Input: part model. Units: mm. Frame: model coordinates. A direction names the side the tool comes from. Round coordinates to 2 decimals unless told otherwise and drop trailing zeros. Loops run counter-clockwise (first coordinate to the right, second up) from the corner with the lowest first, then second, coordinate; pieces in that order, holes last. Notation, with made-up numbers: M -3.5,83.5 L 32.5,83.5 A31 ccw 32.5,119.5 Z; hole C 30,35 d10. An arc over 180 degrees is marked long. Put each result on its own line as item: value. Start each with the question number.
1) Pin query (flat end, axial travel): pin 1 (1.4 mm diameter, centred on x = -45.72, y = -33.02, fed in from +Z); pin 2 (3.5 mm diameter, centred on x = 45, y = 31.5, fed in from +Z); pin 3 (2.5 mm diameter, centred on x = -14.5, z = 28.5, fed in from -Y). Return the tip coordinate at first contact, or that it passes through.
2) Section C-C on z = 22.5. Output: boundary loops of the cut face in (x, y), plus the area to 3 significant figures.
3) Section B-B on z = 4. State how many separate pieces and enclosed holes the cut face has, plus the area to 3 significant figures.
4) Line query: probe 1 along Y at (x, z) = (-45.72, 3.2); probe 2 along Y at (x, z) = (4, 14.25); probe 3 along X at (y, z) = (-13.5, 11.5). Output: solid intervals per line, ascending.
5) Draft query along Z for faces 1 (the face through (-22.2, -41.23, 15.86)), 2 (the face through (52.5, 1, 9)), 3 (the face through (-1, 1, 0)), 4 (the face through (54, 0, 17)). Return one class per face: +Z half, -Z half, draft (parallel to the pull), parting line (faces both ways), or undercut.
6) Reachability of faces 5 (the face through (-1, 40, 14)), 6 (the face through (54, -12.7, 14)), 7 (the face through (-11, -41, 15)) from +Z, -Z, +X, -X, +Y, -Y: full face, straight path, thin tool, end or side. Return the list, or none.
7) Section D-D on x = -12.5. Output: boundary loops of the cut face in (y, z).
8) Section A-A on y = -7. Output: boundary loops of the cut face in (x, z), plus the area to 4 significant figures.
Autodesk Inventor part; units mm, degrees
ref_plane "YZ Plane" through (0, 0, 0) normal (1, 0, 0) x (0, 1, 0)
ref_plane "XZ Plane" through (0, 0, 0) normal (0, 1, 0) x (-1, 0, 0)
ref_plane "XY Plane" through (0, 0, 0) normal (0, 0, 1) x (1, 0, 0)
sketch "Esboço1" plane through (0, 0, 0) normal (0, 0, 1) x (1, 0, 0)
  line L0 (-55, -42.5) -> (55, -42.5)
  line L1 (55, -42.5) -> (55, 42.5)
  line L2 (55, 42.5) -> (-55, 42.5)
  line L3 (-55, 42.5) -> (-55, -42.5)
  line L4 (-55, -42.5) -> (55, 42.5) construction
  line L5 (55, -42.5) -> (-55, 42.5) construction
  point P0 (0, 0)
  dimension "d0" = 110
  dimension "d1" = 85
extrude "Extrusão1" add sketch "Esboço1" along normal blind 2
sketch "Esboço2" plane through (0, 0, 2) normal (0, 0, 1) x (1, 0, 0)
  line L0 (55, 42.5) -> (-55, 42.5)
  line L1 (55, -42.5) -> (-55, -42.5)
  line L2 (-55, -42.5) -> (-55, 42.5)
  line L3 (-55, 42.5) -> (55, 42.5)
  line L4 (55, 42.5) -> (55, -42.5)
  line L5 (55, -42.5) -> (-55, 42.5) construction
  line L6 (-55, -42.5) -> (55, 42.5) construction
  line L7 (52.5, -40) -> (-52.5, -40)
  line L8 (-52.5, -40) -> (-52.5, 40)
  line L9 (-52.5, 40) -> (52.5, 40)
  line L10 (52.5, 40) -> (52.5, -40)
  line L11 (52.5, -40) -> (-52.5, 40) construction
  line L12 (-52.5, -40) -> (52.5, 40) construction
  point P0 (0, 0)
  point P1 (55, 42.5)
  dimension "d4" = 105
  dimension "d5" = 80
extrude "Extrusão2" add sketch "Esboço2" along normal blind 25
sketch "Esboço3" plane through (0, 0, 2) normal (0, 0, 1) x (1, 0, 0)
  line L0 (-45.72, -33.02) -> (45.72, 33.02) construction
  line L1 (45.72, -33.02) -> (-45.72, 33.02) construction
  circle A0 centre (-45.72, 33.02) radius 3.5
  circle A1 centre (45.72, 33.02) radius 3.5
  circle A2 centre (-45.72, -33.02) radius 3.5
  circle A3 centre (45.72, -33.02) radius 3.5
  circle A4 centre (-45.72, 33.02) radius 0.75
  circle A5 centre (45.72, 33.02) radius 0.75
  circle A6 centre (-45.72, -33.02) radius 0.75
  circle A7 centre (45.72, -33.02) radius 0.75
  point P0 (0, 0)
  dimension "d10" = 7
  dimension "d11" = 7
  dimension "d12" = 7
  dimension "d13" = 7
  dimension "d20" = 1.5
  dimension "d21" = 1.5
  dimension "d22" = 1.5
  dimension "d23" = 1.5
extrude "Extrusão3" add sketch "Esboço3" along normal blind 5
sketch "Esboço4" plane through (0, 0, 27) normal (0, 0, 1) x (1, 0, 0)
  line L0 (55, -42.5) -> (-55, -42.5)
  line L1 (-55, -42.5) -> (-55, 42.5)
  line L2 (-55, 42.5) -> (55, 42.5)
  line L3 (55, 42.5) -> (55, -42.5)
  line L4 (55, -42.5) -> (-55, 42.5) construction
  line L5 (-55, -42.5) -> (55, 42.5) construction
  line L6 (54, -41.5) -> (-54, -41.5)
  line L7 (-54, -41.5) -> (-54, 41.5)
  line L8 (-54, 41.5) -> (54, 41.5)
  line L9 (54, 41.5) -> (54, -41.5)
  line L10 (54, -41.5) -> (-54, 41.5) construction
  line L11 (-54, -41.5) -> (54, 41.5) construction
  point P0 (0, 0)
  dimension "d16" = 108
  dimension "d17" = 83
extrude "Extrusão4" add sketch "Esboço4" along normal blind 3
sketch "Esboço8" plane through (-55, -42.5, 0) normal (0, -1, 0) x (1, 0, 0)
  line L0 (31.9, 15) -> (57.3, 15)
  line L1 (57.3, 15) -> (57.3, 30)
  line L2 (57.3, 30) -> (31.9, 30)
  line L3 (31.9, 30) -> (31.9, 15)
  line L4 (0, 30) -> (110, 30)
  line L5 (0, 0) -> (0, 30)
  point P0 (53.5, 0)
  dimension "d55" = 25.4
  dimension "d56" = 15
  dimension "d57" = 31.9
extrude "Extrusão5" cut sketch "Esboço8" against normal blind 3
fillet "Arredondamento5" radius 3 2 edges at (-23.1, -41.25, 15) (2.3, -41.25, 15)
sketch "Esboço11" plane through (55, -42.5, 0) normal (1, 0, 0) x (0, 0, -1)
  line L0 (-30, 0) -> (-30, 85)
  line L1 (0, 0) -> (-30, 0)
  point P0 (0, 42.5)
  point P1 (-22.5, 10)
  dimension "d66" = 7.5
  dimension "d67" = 10
hole "Furo1" at (55, -32.5, 22.5) direction (-1, 0, 0) diameter 7 depth 2.5
sketch "Esboço12" plane through (55, -42.5, 0) normal (1, 0, 0) x (0, 0, -1)
  line L0 (-17, 29.8) -> (-10, 29.8)
  line L1 (-10, 29.8) -> (-10, 55.2)
  line L2 (-10, 55.2) -> (-17, 55.2)
  line L3 (-17, 55.2) -> (-17, 29.8)
  line L4 (0, 0) -> (-30, 0)
  line L5 (0, 0) -> (0, 85)
  point P0 (0, 42.5)
  point P1 (-13.5, 29.8)
  point P2 (-10, 42.5)
  point P3 (0, 42.5)
  dimension "d68" = 7
  dimension "d69" = 25.4
  dimension "d71" = 10
extrude "Extrusão8" cut sketch "Esboço12" against normal blind 3
fillet "Arredondamento6" radius 2 4 edges at (53.75, -12.7, 10) (53.75, -12.7, 17) (53.75, 12.7, 17) (53.75, 12.7, 10)
properties part number "Case" material "ABS plástico"
Geometry results:
1. pin 1: stops at z = 2
1. pin 2: stops at z = 7
1. pin 3: stops at y = 41.5
2. outline: M -55,-42.5 L -23.1,-42.5 L -23.1,-40 L -52.5,-40 L -52.5,40 L 52.5,40 L 52.5,-29 L 55,-29 L 55,42.5 L -55,42.5 Z; M 2.3,-42.5 L 55,-42.5 L 55,-36 L 52.5,-36 L 52.5,-40 L 2.3,-40 Z
2. area: 869 mm²
3. separate pieces: 5
3. enclosed holes: 5
3. area: 1,100 mm²
4. probe 1: y = -42.5 to -40, -36.52 to -33.77, -32.27 to -29.52, 29.52 to 32.27, 33.77 to 36.52, 40 to 42.5
4. probe 2: y = -42.5 to -40, 40 to 42.5
4. probe 3: x = -55 to -52.5, 52.5 to 55
5. face 1: +Z half
5. face 2: draft
5. face 3: -Z half
5. face 4: undercut
6. face 5: +Z
6. face 6: +X
6. face 7: +Z, -Y
7. outline: M -42.5,0 L 42.5,0 L 42.5,30 L 41.5,30 L 41.5,27 L 40,27 L 40,2 L -40,2 L -40,15 L -42.5,15 Z
8. outline: M -55,0 L 55,0 L 55,10 L 52.5,10 L 52.5,2 L -52.5,2 L -52.5,27 L -54,27 L -54,30 L -55,30 Z; M 52.5,17 L 55,17 L 55,30 L 54,30 L 54,27 L 52.5,27 Z
8. area: 333.5 mm²
